Can you work these out from the model? Positions are in its coordinate system, mm. A direction names the side the tool comes from. Coordinates: 2 decimals unless noted, no trailing zeros. Order: outer loops, then holes, each group sorted by start corner. A loop starts at its lowest first (then second) coordinate and runs counter-clockwise, first axis right, second up. Notation, with made-up numbers: (37, 33.25) -> (59, 33.25) arc R15 ccw to (59, 40.25) -> close; hole circle Ø10 at (-28, -14.5). An arc over 180 degrees is marked (long way). Use a Markdown table: item, result. Add a question column.
1. For pin 1 Ø10 at (x, z) = (65.5, 5.5) entering from -Y; pin 2 Ø11 at (y, z) = (-18, 34) entering from +X; pin 3 Ø1 at (y, z) = (11.5, 11) entering from +X; pin 4 Ø24 at (x, y) = (0, 0) entering from -Z, each with a flat end and sliding along its axis, tell me the tip position at first contact or that it passes through.
2. For faces 4 (the flat face through (17, 10, 30)), 5 (the flat face through (60.576, -19.766, 4.951)), 6 (the flat face through (-5, -19, 35)), which set-ups out of +Z, -Z, +X, -X, +Y, -Y let a thin tool reach every point of the face, with its end or its side?
3. Suppose I cut it at A-A, the plane x = 0. List the corners of the cut face in (y, z) for me, then the cut area to 4 significant figures.
4. Suppose I cut it at C-C, the plane z = 35. List the corners of the cut face in (x, y) for me, then the cut area to 3 significant figures.
5. If I drill on line 1 along Y through (x, z) = (0, 17); line 2 along X through (y, z) = (11.5, 33); line 3 along X through (y, z) = (-18.5, 37.5), over which ranges is the centre line in solid material (lowest first)? Write a range as from..to.
6. We'd pull the mould along X, two halves only. Please class faces 1 (the flat face through (-14.168, 13.953, 34.93)), 2 (the cylindrical face through (92.566, 53.705, 4.93)), 3 (the flat face through (19.168, 5.293, 34.93)): pulls with the +X half, pulls with the -X half, needs draft (parallel to the pull), parting line crosses it, or undercut.
7. Suppose I cut it at B-B, the plane x = 80. List the corners of the cut face in (y, z) for me.
8. Suppose I cut it at D-D, the plane z = 21.5. List the corners of the cut face in (x, y) for me.
Autodesk Inventor part; units mm, degrees
ref_plane "YZ Plane" through (0, 0, 0) normal (1, 0, 0) x (0, 1, 0)
ref_plane "XZ Plane" through (0, 0, 0) normal (0, 1, 0) x (-1, 0, 0)
ref_plane "XY Plane" through (0, 0, 0) normal (0, 0, 1) x (1, 0, 0)
sketch "Sketch1" plane through (0, 0, 0) normal (0, 0, 1) x (1, 0, 0)
  arc A0 (8.0041, 44.2824) -> (7.8263, -44.3142) centre (0, 0) ccw
  arc A1 (8.0041, 44.2824) -> (66.8467, 56.6014) centre (22.2337, 123.0068) ccw
  arc A2 (93.3944, 27.2324) -> (66.8467, 56.6014) centre (78, 40) ccw
  arc A3 (89.7392, -29.8476) -> (95.1215, -12.9797) centre (88, -20) ccw
  arc A4 (93.3944, 27.2324) -> (95.1215, -12.9797) centre (116.4861, 8.081) ccw
  line L0 (7.8263, -44.3142) -> (89.7392, -29.8476)
  circle A5 centre (78, 40) radius 10
  arc A6 (70.8456, 19.3234) -> (42.1311, 16.5) centre (56.0864, 22) ccw
  arc A7 (43.9366, -10.8099) -> (53.0508, -21.095) centre (51.5602, -13.2351) ccw
  line L1 (53.0508, -21.095) -> (68.3146, -18.3992)
  arc A8 (68.3146, -18.3992) -> (74.1186, -7.243) centre (66.8289, -10.5384) ccw
  arc A9 (70.8456, 19.3234) -> (74.1186, -7.243) centre (115.1234, 11.2936) ccw
  arc A10 (8.0041, 44.2824) -> (7.8263, -44.3142) centre (0, 0) ccw
  arc A11 (43.9366, -10.8099) -> (42.1311, 16.5) centre (0, 0) ccw
  circle A12 centre (0, 35) radius 5
  line L2 (0, 0) -> (35, 0) construction
  circle A13 centre (-24.7487, -24.7487) radius 5
  circle A14 centre (24.7487, -24.7487) radius 5
  dimension "d1" = 160
  dimension "d2" = 40
  dimension "d3" = 40
  dimension "d4" = 78
  dimension "d6" = 20
  dimension "d7" = 88
  dimension "d8" = 20
  dimension "d9" = 60
  dimension "d10" = 20
  dimension "d12" = 30
  dimension "d13" = 22
  dimension "d22" = 16
  dimension "d23" = 15.5
  dimension "d26" = 90
  dimension "d29" = 10
  dimension "d32" = 10
  dimension "d33" = 10
  dimension "d76" = 15
extrude "Extrusion1" add sketch "Sketch1" along normal blind 10
sketch "Sketch2" plane through (0, 0, 10) normal (0, 0, 1) x (1, 0, 0)
  circle A0 centre (0, 0) radius 25
  circle A1 centre (0, 0) radius 15
  line L0 (0, 0) -> (25, 0) construction
  line L1 (0, 0) -> (25, 0) construction
  line L2 (-5, -15) -> (-5, -24.4949)
  line L3 (5, -24.4949) -> (5, -15)
  line L4 (-5, -15) -> (-5, -14.1421)
  line L5 (5, -15) -> (5, -14.1421)
  line L6 (0, 0) -> (30, 0) construction
  line L7 (0, 0) -> (30, 0) construction
  line L8 (-23.7132, 7.9173) -> (-14.7474, 2.7409)
  line L9 (-9.7474, 11.4012) -> (-18.7132, 16.5776)
  line L10 (18.7132, 16.5776) -> (9.7474, 11.4012)
  line L11 (14.7474, 2.7409) -> (23.7132, 7.9173)
  dimension "d36" = 50
  dimension "d37" = 30
  dimension "d59" = 10
extrude "Extrusion2" add sketch "Sketch2" along normal blind 30 contours A0 L3 L5 A1 L11 | L10 A1 L9 A0 | A0 L8 A1 L4 L2
chamfer "Chamfer1" distance 0.5 angle 45 6 edges at (-29.7487, -24.7487, 10) (-5, 35, 10) (19.7487, -24.7487, 0) (19.7487, -24.7487, 10) (-29.7487, -24.7487, 0) (-5, 35, 0)
chamfer "Chamfer2" distance 1.5 angle 45 6 edges at (45.5728, -18.5409, 0) (45.1483, 2.9848, 0) (54.6186, 36.928, 0) (70.4611, 5.7912, 0) (73.9259, -14.2306, 0) (60.6827, -19.7471, 0)
sketch "Sketch3" plane through (0, 0, 10) normal (0, 0, 1) x (1, 0, 0)
  line L0 (23.7132, 7.9173) -> (14.7474, 2.7409)
  circle A0 centre (0, 0) radius 25
  circle A1 centre (0, 0) radius 15
  line L1 (9.7474, 11.4012) -> (18.7132, 16.5776)
  line L2 (9.7474, 11.4012) -> (18.7132, 16.5776)
  line L3 (14.7474, 2.7409) -> (23.7132, 7.9173)
  line L4 (5, -14.1421) -> (5, -24.4949)
  line L5 (-5, -24.4949) -> (-5, -14.1421)
  line L6 (-5, -14.1421) -> (-5, -24.4949)
  line L7 (-14.7474, 2.7409) -> (-23.7132, 7.9173)
  line L8 (-23.7132, 7.9173) -> (-14.7474, 2.7409)
  line L9 (-18.7132, 16.5776) -> (-9.7474, 11.4012)
  line L10 (-18.7132, 16.5776) -> (-9.7474, 11.4012)
extrude "Extrusion3" add sketch "Sketch3" along normal blind 20 contours L0 A1 L1 A0 | A0 L5 A1 L4 | L9 A1 L7 A0
sketch "Sketch4" plane through (0, 0, 10) normal (0, 0, 1) x (1, 0, 0)
  circle A0 centre (0, 0) radius 15
extrude "Extrusion4" cut sketch "Sketch4" against normal blind 10
thread "Thread1"
thread "Thread2"
thread "Thread3"
chamfer "Chamfer4" distance 1.5 angle 45 6 edges at (54.6186, 36.928, 10) (70.4611, 5.7912, 10) (73.9259, -14.2306, 10) (45.1483, 2.9848, 10) (45.5728, -18.5409, 10) (60.6827, -19.7471, 10)
properties part number "Curved Disc new" material "Steel, Mild, Welded"
Worked out:
| question | item | result |
|---|---|---|
| 1 | pin 1 | stops at y = -35.01 |
| 1 | pin 2 | stops at x = 21.65 |
| 1 | pin 3 | stops at x = 22.45 |
| 1 | pin 4 | passes through |
| 2 | face 4 | +Z |
| 2 | face 5 | +Z, -Z |
| 2 | face 6 | +Z, -Y |
| 3 | outline | (-45, 0) -> (-15, 0) -> (-15, 30) -> (-25, 30) -> (-25, 10) -> (-45, 10) -> close; (15, 0) -> (29.5, 0) -> (30, 0.5) -> (30, 9.5) -> (29.5, 10) -> (25, 10) -> (25, 40) -> (15, 40) -> close; (40, 0.5) -> (40.5, 0) -> (45, 0) -> (45, 10) -> (40.5, 10) -> (40, 9.5) -> close |
| 3 | area | 999.5 mm² |
| 4 | outline | (-23.71, 7.92) arc R25 ccw to (-5, -24.49) -> (-5, -14.14) arc R15 cw to (-14.75, 2.74) -> close; (-18.71, 16.58) -> (-9.75, 11.4) arc R15 cw to (9.75, 11.4) -> (18.71, 16.58) arc R25 ccw to start; (5, -24.49) arc R25 ccw to (23.71, 7.92) -> (14.75, 2.74) arc R15 cw to (5, -14.14) -> close |
| 4 | area | 953 mm² |
| 5 | line 1 | y = -25..-15, 15..25 |
| 5 | line 2 | x = -9.92..-9.63, 9.63..9.92 |
| 5 | line 3 | x = -16.82..-5, 5..16.82 |
| 6 | face 1 | pulls with the -X half |
| 6 | face 2 | parting line crosses it |
| 6 | face 3 | undercut |
| 7 | outline | (-31.57, 0) -> (30.2, 0) -> (30.2, 10) -> (-31.57, 10) -> close; (49.8, 0) -> (59.9, 0) -> (59.9, 10) -> (49.8, 10) -> close |
| 8 | outline | circle Ø50 at (0, 0); hole circle Ø30 at (0, 0) |
